Can you work these out from the model? Positions are in its coordinate system, mm. Face numbers are marked on the shaded views. A direction names the side the tool comes from. Coordinates: 2 decimals unless noted, no trailing zeros. Write each loop counter-clockwise with the first axis right and the second up, starting at its lowest first coordinate (ties: lowest second). Pieces come first, ordered by that corner, then holes.
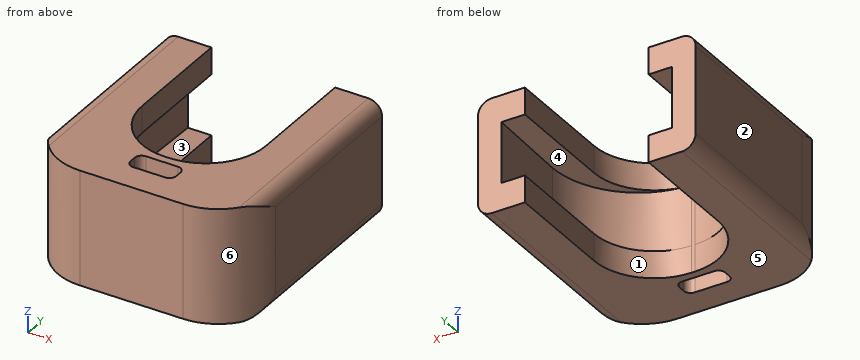
```python
from build123d import *

# Parameters (mm, degrees)
SKETCH1_W                      = 24.13
SKETCH1_H                      = 12.7
BOSS_EXTRUDE1_DEPTH            = 25.4
CUT_EXTRUDE2_DEPTH             = 19.05
FILLET1_R                      = 9.525
FILLET2_R                      = 6.6675
BOSS_EXTRUDE2_DEPTH            = 3.3655
CUT_EXTRUDE3_REACH             = 39.265
SKETCH4_W                      = 5.08
SKETCH4_H                      = 2.286
CUT_EXTRUDE3_DIRECTION_2_DEPTH = 38.265357908
FILLET3_R                      = 0.762
FILLET4_R                      = 1.524
FILLET5_R                      = 6.35


# Some blends are built 0.0001 mm under size
with BuildPart() as part:
    # Sketch1 → Boss-Extrude1 (new body)
    with BuildSketch(Plane(origin=(0, 0, 0), x_dir=(1, 0, 0), z_dir=(0, 1, 0))):
        with Locations((12.065, 6.35)):
            Rectangle(SKETCH1_W, SKETCH1_H)
    extrude(amount=BOSS_EXTRUDE1_DEPTH)

    # Sketch2 → Cut-Extrude2 (cut)
    with BuildSketch(Plane(origin=(0, 25.4, 0), x_dir=(1, 0, 0), z_dir=(0, 1, 0))):
        Polygon((2.3495, 2.9845), (5.207, 2.9845), (5.207, 0), (18.923, 0), (18.923, 2.9845), (21.7805, 2.9845), (21.7805, 9.7155), (18.923, 9.7155), (18.923, 12.7), (5.207, 12.7), (5.207, 9.7155), (2.3495, 9.7155), align=None)
    extrude(amount=-CUT_EXTRUDE2_DEPTH, mode=Mode.SUBTRACT)

    # Fillet1
    fillet1_edges = [part.edges().sort_by_distance(p)[0] for p in [
        (21.7805, 6.35, -6.35),
        (2.3495, 6.35, -6.35),
    ]]
    fillet(fillet1_edges, radius=FILLET1_R)

    # Fillet2
    fillet2_edges = [part.edges().sort_by_distance(p)[0] for p in [
        (5.207, 9.072789422, -11.20775),
        (18.923, 9.072789422, -11.20775),
        (18.923, 9.072789422, -1.49225),
        (5.207, 9.072789422, -1.49225),
    ]]
    fillet(fillet2_edges, radius=FILLET2_R - 0.0001)  # a hair under: the kernel refuses the full size

    # Sketch3 → Boss-Extrude2 (add, symmetric)
    with BuildSketch(Plane.XY.offset(-6.35)):
        Polygon((21.7805, 25.4), (21.5265, 25.4), (21.7805, 15.875), align=None)
        Polygon((2.3495, 25.4), (2.6035, 25.4), (2.3495, 15.875), align=None)
    extrude(amount=BOSS_EXTRUDE2_DEPTH, both=True)

    # Sketch4 → Cut-Extrude3 (cut, up to next)
    with BuildSketch(Plane.XY, mode=Mode.PRIVATE) as cut_extrude3_sk1:
        with Locations((12.065, 4.318)):
            Rectangle(SKETCH4_W, SKETCH4_H)
    cut_extrude3_tool1 = extrude(cut_extrude3_sk1.sketch, amount=-CUT_EXTRUDE3_REACH, mode=Mode.PRIVATE) & part.part
    add(cut_extrude3_tool1.solids().sort_by_distance((12.065, 4.318, 0))[0], mode=Mode.SUBTRACT)

    # Sketch4 → Cut-Extrude3 direction 2 (cut)
    with BuildSketch(Plane.XY):
        with Locations((12.065, 4.318)):
            Rectangle(SKETCH4_W, SKETCH4_H)
    extrude(amount=CUT_EXTRUDE3_DIRECTION_2_DEPTH, mode=Mode.SUBTRACT)

    # Fillet3
    fillet3_edges = [part.edges().sort_by_distance(p)[0] for p in [
        (9.525, 5.461, -6.35),
        (9.525, 3.175, -6.35),
        (14.605, 3.175, -6.35),
        (14.605, 5.461, -6.35),
    ]]
    fillet(fillet3_edges, radius=FILLET3_R)

    # Fillet4
    fillet4_edges = [part.edges().sort_by_distance(p)[0] for p in [
        (0, 12.7, -12.7),
        (24.13, 12.7, -12.7),
        (24.13, 12.7, 0),
        (0, 12.7, 0),
    ]]
    fillet(fillet4_edges, radius=FILLET4_R)

    # Fillet5
    # the kernel refuses this fillet: 6.35 mm, written as the material it takes off along each edge
    with BuildSketch(Plane(origin=(24.13, 0, 14.351), x_dir=(-1, 0, 0), z_dir=(0, 0, -1)), Plane(origin=(0, 0, -27.051), x_dir=(1, 0, 0), z_dir=(0, 0, 1))) as fillet5_piece_1:
        with BuildLine():
            CenterArc((FILLET5_R, FILLET5_R), FILLET5_R, 180, 90)
            Line((0, FILLET5_R), (0, 0))
            Line((0, 0), (FILLET5_R, 0))
        make_face()
    extrude(amount=41.402, mode=Mode.SUBTRACT)


solid = part.part
```
1. If we section it at C-C, the plane x = 17: List the corners of the cut face in (y, z) for me.
2. We'd pull the mould along Z, two halves only. Please class the marked faces 3, 4, 5 and 6: released by +Z, released by -Z, zero draft, split by the parting line, or undercut.
3. I'm going to push flat-ended pins straight in: P1, Ø1.5, axis at y = 17.5, z = -1, coming from the +X side; P2, Ø3, axis at x = 12.5, z = -4.5, coming from the +Y side. Where does each tip first touch, or does it pass through?
4. Which directions (+Z, -Z, +X, -X, +Y, -Y) give clear straight access to the entire face, cutting with the end or side of a thin tool? Please do the marked faces 1 and 2.
5. If I drill on L1, parallel to Y at x = 12, z = -9 (3 decimals); L2, parallel to Z at x = 16.5, y = 7.75; L3, parallel to X at y = 16.5, z = -9.75, over which ranges is the centre line in solid material (lowest first)?
6. If we section it at D-D, the plane y = 15: List the corners of the cut face in (x, z) for me.
7. If we section it at B-B, the plane y = 3.5: List the corners of the cut face in (x, z) for me.
Answers:
1. outline: (0, -12.7) - (8.33, -12.7) - (8.33, -9.72) - (7.62, -9.72) - (7.62, -2.98) - (8.33, -2.98) - (8.33, 0) - (0, 0) - close
2. face 3: undercut
2. face 4: undercut
2. face 5: released by -Z
2. face 6: zero draft
3. P1: stops at x = 24.13
3. P2: stops at y = 6.51
4. face 1: +Z, -Z, +Y
4. face 2: +Z, -Z, -X, +Y, -Y
5. L1: y = 0 to 3.175, 5.461 to 6.35
5. L2: z = -12.7 to -9.72, -2.98 to 0
5. L3: x = 0 to 5.21, 18.92 to 24.13
6. outline: (0, -11.18) arc R1.52 ccw to (1.52, -12.7) - (5.21, -12.7) - (5.21, -9.72) - (2.39, -9.72) - (2.39, -2.98) - (5.21, -2.98) - (5.21, 0) - (1.52, 0) arc R1.52 ccw to (0, -1.52) - close; (18.92, -12.7) - (22.61, -12.7) arc R1.52 ccw to (24.13, -11.18) - (24.13, -1.52) arc R1.52 ccw to (22.61, 0) - (18.92, 0) - (18.92, -2.98) - (21.74, -2.98) - (21.74, -9.72) - (18.92, -9.72) - close
7. outline: (0.68, -12.44) arc R1.52 ccw to (1.52, -12.7) - (9.66, -12.7) - (9.66, 0) - (1.52, 0) arc R1.52 ccw to (0.68, -0.26) - close; (14.47, -12.7) - (22.61, -12.7) arc R1.52 ccw to (23.45, -12.44) - (23.45, -0.26) arc R1.52 ccw to (22.61, 0) - (14.47, 0) - close
